The model under review builds one solid part; all positions refer to its coordinate system, in mm. Face numbers are marked on the shaded views. Round coordinates to 2 decimals unless told otherwise and drop trailing zeros. Order: outer loops, then holes, each group sorted by start corner. A loop starts at its lowest first (then second) coordinate and runs counter-clockwise, first axis right, second up. Notation, with made-up numbers: (26, 73.25) -> (59, 73.25) arc R23 ccw to (59, 104.25) -> close; hole circle Ø10 at (15, 59). An arc over 180 degrees is marked (long way). Use a Markdown table: item, result. Add a question column.
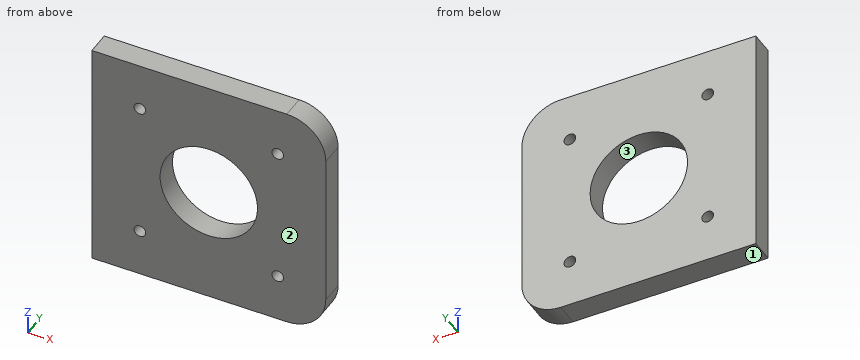
```python
from build123d import *

# Parameters (mm, degrees)
SKETCH1_W           = 60
SKETCH1_H           = 60
SKETCH1_R           = 1.5
SKETCH1_R_2         = 12.5
BOSS_EXTRUDE1_DEPTH = 6
FILLET1_R           = 10
SCALE2_SCALE        = 7.5


with BuildPart() as part:
    # Sketch1 → Boss-Extrude1 (new body)
    with BuildSketch(Plane(origin=(0, 0, 0), x_dir=(1, 0, 0), z_dir=(0, 1, 0))):
        with Locations((17.68, 17.68)):
            Rectangle(SKETCH1_W, SKETCH1_H)
        with Locations((0, 35.36)):
            Circle(SKETCH1_R, mode=Mode.SUBTRACT)
        with Locations((35.36, 35.36)):
            Circle(SKETCH1_R, mode=Mode.SUBTRACT)
        with Locations((35.36, 0)):
            Circle(SKETCH1_R, mode=Mode.SUBTRACT)
        Circle(SKETCH1_R, mode=Mode.SUBTRACT)
        with Locations((17.68, 17.68)):
            Circle(SKETCH1_R_2, mode=Mode.SUBTRACT)
    extrude(amount=BOSS_EXTRUDE1_DEPTH)

    # Fillet1
    fillet1_edges = [part.edges().sort_by_distance(p)[0] for p in [
        (47.68, 3, -47.68),
        (47.68, 3, 12.32),
    ]]
    fillet(fillet1_edges, radius=FILLET1_R)


with BuildPart() as part_1:
    # Scale2: scaled about (17.28771311, 3, -17.68)
    add(part.part.scale(SCALE2_SCALE).moved(Location((-112.370135215, -19.5, 114.92))))


solid = part_1.part
```
Q1. Add section D-D, the plane z = -150.28. Give the boundary of the cut face in (x, y).
Q2. To check wall thickness, follow line 1 along X through (y, z) = (7, 114.92); line 2 along X through (y, z) = (-9, 114); line 3 along Z through (x, y) = (-122.5, 3.5). State the ranges of each line that lie inside material, in increasing order.
Q3. Add section B-B, the plane y = 5. Give the boundary of the cut face in (x, z), then the cut area to 3 significant figures.
Q4. Draft analysis for pull direction Z (two halves, no side actions). For the marked faces 1, 2 and 3, state which applies: released by +Z, released by -Z, zero draft, split by the parting line, or undercut.
Q5. For pin 1 (13.5 mm diameter, centred on x = 152.83, z = 114.92, fed in from +Y); pin 2 (1 mm diameter, centred on y = -0.5, z = 159, fed in from +X), all flat-tipped, find the tip position at first contact; note any pin that passes through.
Q6. Add section C-C, the plane x = 80. Give the boundary of the cut face in (y, z), then the cut area to 3 significant figures.
Q7. Add section A-A, the plane z = -17.68. Give the boundary of the cut face in (x, y), then the cut area to 3 significant figures.
Return value:
| question | item | result |
|---|---|---|
| 1 | outline | (-204.77, -19.5) -> (-123.62, -19.5) -> (-123.62, 25.5) -> (-204.77, 25.5) -> close; (-101.12, -19.5) -> (141.58, -19.5) -> (141.58, 25.5) -> (-101.12, 25.5) -> close; (164.08, -19.5) -> (245.23, -19.5) -> (245.23, 25.5) -> (164.08, 25.5) -> close |
| 2 | line 1 | -204.77 to -123.62, -101.12 to 141.58, 164.08 to 245.23 |
| 2 | line 2 | -204.77 to -123.58, -101.16 to 141.62, 164.04 to 245.23 |
| 2 | line 3 | -242.68 to -155.17, -145.39 to 110.03, 119.81 to 207.32 |
| 3 | outline | (-204.77, -242.68) -> (170.23, -242.68) arc R75 ccw to (245.23, -167.68) -> (245.23, 132.32) arc R75 ccw to (170.23, 207.32) -> (-204.77, 207.32) -> close; hole circle Ø22.5 at (-112.37, -150.28); hole circle Ø22.5 at (-112.37, 114.92); hole circle Ø187.5 at (20.23, -17.68); hole circle Ø22.5 at (152.83, -150.28); hole circle Ø22.5 at (152.83, 114.92) |
| 3 | area | 171,000 mm² |
| 4 | face 1 | released by -Z |
| 4 | face 2 | zero draft |
| 4 | face 3 | undercut |
| 5 | pin 1 | through |
| 5 | pin 2 | x = 240.51 |
| 6 | outline | (-19.5, -242.68) -> (25.5, -242.68) -> (25.5, -89.91) -> (-19.5, -89.91) -> close; (-19.5, 54.55) -> (25.5, 54.55) -> (25.5, 207.32) -> (-19.5, 207.32) -> close |
| 6 | area | 13,700 mm² |
| 7 | outline | (-204.77, -19.5) -> (-73.52, -19.5) -> (-73.52, 25.5) -> (-204.77, 25.5) -> close; (113.98, -19.5) -> (245.23, -19.5) -> (245.23, 25.5) -> (113.98, 25.5) -> close |
| 7 | area | 11,800 mm² |
